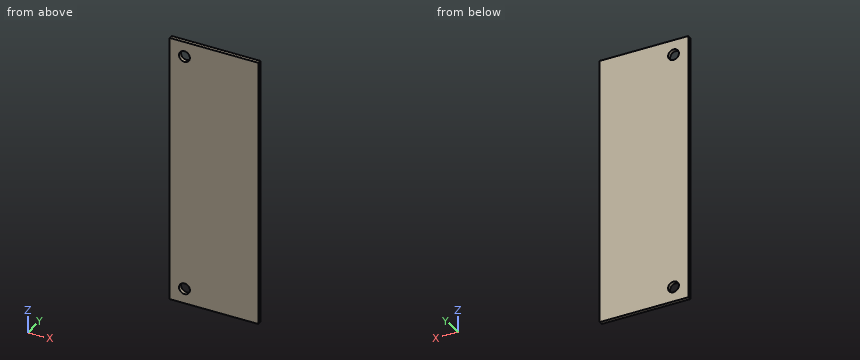
Autodesk Inventor part; units mm, degrees
ref_plane "YZ Plane" through (0, 0, 0) normal (1, 0, 0) x (0, 1, 0)
ref_plane "XZ Plane" through (0, 0, 0) normal (0, 1, 0) x (-1, 0, 0)
ref_plane "XY Plane" through (0, 0, 0) normal (0, 0, 1) x (1, 0, 0)
sketch "Sketch4" plane through (0, 0, 0) normal (0, 1, 0) x (-1, 0, 0)
  line L0 (-6.6563, 17.1443) -> (-44.7563, 17.1443)
  line L1 (-44.7563, 17.1443) -> (-44.7563, -97.1557)
  line L2 (-44.7563, -97.1557) -> (-6.6563, -97.1557)
  line L3 (-6.6563, -97.1557) -> (-6.6563, 17.1443)
  circle A0 centre (-13.0063, 10.7943) radius 2.3368
  circle A1 centre (-13.0063, -90.8057) radius 2.3368
  point P0 (0, 0)
  dimension "d41" = 38.1
  dimension "d42" = 114.3
  dimension "d43" = 4.6736
  dimension "d44" = 4.6736
  dimension "d45" = 6.35
  dimension "d46" = 6.35
  dimension "d47" = 6.35
  dimension "d48" = 6.35
extrude "Plate4" add sketch "Sketch4" along normal blind 1.5875
equation "\"d49\" = Thickness"
equation "\"BendRadius\" = Thickness"
equation "\"BendReliefWidth\" = Thickness"
equation "\"BendReliefDepth\" = 0.5 * Thickness"
equation "\"CornerReliefSize\" = 4 * Thickness"
equation "\"MinimumRemnant\" = 2 * Thickness"
equation "\"TransitionRadius\" = BendRadius"
equation "\"JacobiRadiusSize\" = BendRadius"
equation "\"GapSize\" = Thickness"
properties part number "underside"
Work out the finished part from the listing and answer in its coordinate system (mm). Round coordinates to 2 decimals unless told otherwise and drop trailing zeros. Write each loop counter-clockwise with the first axis right and the second up, starting at its lowest first coordinate (ties: lowest second). Pieces come first, ordered by that corner, then holes.
1) A cutting plane is placed at A-A on x = 13.5. Determine the outline of the cut face in (y, z), and give its area (3 significant figures).
2) Consider probe 1 along X at (y, z) = (1.35, -90); probe 2 along X at (y, z) = (1.1, 12.5). Determine where each line is inside the solid, lowest interval first.
3) A flat-ended cylindrical pin translates along its axis: P1, Ø5, axis at x = 20.5, z = -72.5, coming from the -Y side. Find the tip coordinate at first contact, or state that the pin passes through.
Entries:
1. outline: (0, -97.16) - (1.59, -97.16) - (1.59, -93.09) - (0, -93.09) - close; (0, -88.52) - (1.59, -88.52) - (1.59, 8.51) - (0, 8.51) - close; (0, 13.08) - (1.59, 13.08) - (1.59, 17.14) - (0, 17.14) - close
1. area: 167 mm2
2. probe 1: x = 6.66 to 10.81, 15.2 to 44.76
2. probe 2: x = 6.66 to 11.41, 14.6 to 44.76
3. P1: stops at y = 0
